from build123d import *

# Parameters (mm, degrees)
BASPROSKE_W         = 4.55
BASPROSKE_H         = 12
TOOTHCUT_DEPTH      = 18.569931702
TEETHCUTS_COUNT     = 22
TEETHCUTS_ANGLE     = 343.636363636
BORSKE_R            = 1.7
BORE_DEPTH          = 50.0000508
SKETCH1_R           = 5
BOSS_EXTRUDE1_DEPTH = 2
CUT_EXTRUDE1_START  = 2
SKETCH1_2_W         = 5
SKETCH1_2_H         = 5
CUT_EXTRUDE1_DEPTH  = 2.55
SKETCH1_4_R         = 6
SKETCH1_4_R_2       = 5
BOSS_EXTRUDE2_DEPTH = 1
CUT_EXTRUDE2_DEPTH  = 2


with BuildPart() as part:
    # BasProSke → Base-Revolve (revolve)
    with BuildSketch(Plane(origin=(0, 0, 0), x_dir=(1, 0, 0), z_dir=(0, 1, 0)), mode=Mode.PRIVATE) as base_revolve_sk:
        with Locations((2.275, 6)):
            Rectangle(BASPROSKE_W, BASPROSKE_H)
    revolve(base_revolve_sk.sketch.rotate(Axis((-10, 0, 0), (1, 0, 0)), 180), axis=Axis((-10, 0, 0), (1, 0, 0)))

    # TooCutSke → ToothCut (cut, through all)
    with BuildSketch(Plane(origin=(0, 0, 0), x_dir=(0, 0, -1), z_dir=(1, 0, 0))):
        with BuildLine():
            ThreePointArc((0.491001901, 9.736627657), (0, 9.749), (-0.491001901, 9.736627657))
            ThreePointArc((-0.491001901, 9.736627657), (-0.822824844, 10.904005344), (-1.46093845, 11.936327074))
            ThreePointArc((-1.46093845, 11.936327074), (0, 12.0254), (1.46093845, 11.936327074))
            ThreePointArc((1.46093845, 11.936327074), (0.822824844, 10.904005344), (0.491001901, 9.736627657))
        make_face()
    toothcut = extrude(amount=TOOTHCUT_DEPTH, mode=Mode.SUBTRACT)

    # TeethCuts: ToothCut ×22 about axis
    teethcuts_axis = Axis((-10, 0, 0), (1, 0, 0))
    for i in range(1, TEETHCUTS_COUNT):
        add(toothcut.rotate(teethcuts_axis, i * TEETHCUTS_ANGLE / (TEETHCUTS_COUNT - 1)), mode=Mode.SUBTRACT)

    # BorSke → Bore (cut, symmetric)
    with BuildSketch(Plane(origin=(0, 0, 0), x_dir=(0, 0, -1), z_dir=(1, 0, 0))):
        with Locations(Location((0, 0, 0), (0, 0, 180))):
            Circle(BORSKE_R)
    extrude(amount=BORE_DEPTH, both=True, mode=Mode.SUBTRACT)

    # Sketch1 → Boss-Extrude1 (add)
    with BuildSketch(Plane.ZY):
        with Locations(Location((0, 0, 0), (0, 0, 180))):
            Circle(SKETCH1_R)
    extrude(amount=BOSS_EXTRUDE1_DEPTH)

    # Sketch1<2> → Cut-Extrude1 (cut)
    with BuildSketch(Plane.ZY.offset(CUT_EXTRUDE1_START)):
        Rectangle(SKETCH1_2_W, SKETCH1_2_H)
    extrude(amount=-CUT_EXTRUDE1_DEPTH, mode=Mode.SUBTRACT)

    # Sketch1<4> → Boss-Extrude2 (add)
    with BuildSketch(Plane.ZY):
        with Locations(Location((0, 0, 0), (0, 0, 180))):
            Circle(SKETCH1_4_R)
        Circle(SKETCH1_4_R_2, mode=Mode.SUBTRACT)
    extrude(amount=BOSS_EXTRUDE2_DEPTH)

    # Sketch2 → Cut-Extrude2 (cut)
    with BuildSketch(Plane(origin=(4.55, 0, 0), x_dir=(0, 0, -1), z_dir=(1, 0, 0))):
        Polygon((1.645448267, 2.85), (-1.645448267, 2.85), (-3.290896534, 0), (-1.645448267, -2.85), (1.645448267, -2.85), (3.290896534, 0), align=None)
    extrude(amount=-CUT_EXTRUDE2_DEPTH, mode=Mode.SUBTRACT)


solid = part.part
Part model, mm, in its own coordinate system. A direction names the side the tool comes from. Round coordinates to 2 decimals unless told otherwise and drop trailing zeros. Loops run counter-clockwise (first coordinate to the right, second up) from the corner with the lowest first, then second, coordinate; pieces in that order, holes last. Notation, with made-up numbers: (62.25, 65.25) - (96.25, 65.25) arc R22 cw to (96.25, 73.25) - close; hole circle Ø6 at (30.5, -33.75). An arc over 180 degrees is marked (long way). Answer as a JSON object with one key per item and string values.
Item 1: Tool access for faces 1 (the face through (4, -2.85, 0)), 2 (the face through (2.24, -10.87, -0.81)), 3 (the face through (2.24, -1.38, 9.65)), 4 (the face through (2.2, -9.6, -5.2)), 5 (the face through (2.24, -7.76, -7.7)): list every direction of +Z, -Z, +X, -X, +Y, -Y with a clear straight run to the whole face (end or side of a thin tool).
Output:
{"face 1": "+X", "face 2": "+X, -X, -Y", "face 3": "+Z, +X, -X", "face 4": "+X, -X", "face 5": "-Z, +X, -X"}
Item 2: Band-saw the part on B-B on z = 10.75. List the corners of the cut face in (x, y).
Output:
{"outline": "(0, -3.76) - (4.55, -3.76) - (4.55, -2.41) - (0, -2.41) - close; (0, -0.78) - (4.55, -0.78) - (4.55, 0.78) - (0, 0.78) - close; (0, 2.41) - (4.55, 2.41) - (4.55, 3.76) - (0, 3.76) - close"}
Item 3: Wall check: L1, parallel to Y at x = 3.75, z = 10.75; L2, parallel to Y at x = 0.75, z = -9; L3, parallel to Z at x = 4, y = 9. Give the ranges that are in metal, low to high.
Output:
{"L1": "-3.76 to -2.41, -0.78 to 0.78, 2.41 to 3.76", "L2": "-6.58 to -4.74, -3.75 to 3.75, 4.74 to 6.58", "L3": "-7.94 to -7.06, -5.06 to 5.06, 7.06 to 7.94"}
Item 4: Pull direction Y, two halves, no side cores. Call faces 6 (the face through (2.24, 8.73, -6.59)), 7 (the face through (2.2, -9.6, 5.2)), 8 (the face through (2.24, -8.71, -6.56)): pulls with the +Y half, pulls with the -Y half, needs draft (parallel to the pull), parting line crosses it, or undercut.
Output:
{"face 6": "pulls with the +Y half", "face 7": "undercut", "face 8": "pulls with the -Y half"}
Item 5: Band-saw the part on A-A on z = 0. List the corners of the cut face in (x, y), plus the area to 3 significant figures.
Output:
{"outline": "(-2, -5) - (-1, -5) - (-1, -6) - (0, -6) - (0, -9.75) - (4.55, -9.75) - (4.55, -2.85) - (2.55, -2.85) - (2.55, -1.7) - (0.55, -1.7) - (0.55, -2.5) - (-2, -2.5) - close; (-2, 2.5) - (0.55, 2.5) - (0.55, 1.7) - (2.55, 1.7) - (2.55, 2.85) - (4.55, 2.85) - (4.55, 9.75) - (0, 9.75) - (0, 6) - (-1, 6) - (-1, 5) - (-2, 5) - close", "area": "79.8 mm2"}
Item 6: Pin check, flat tips, straight feed: pin 1 (2 mm diameter, centred on x = -0.5, z = -0.5, fed in from +Y); pin 2 (1 mm diameter, centred on x = 0, y = -6.5, fed in from +Z); pin 3 (1.5 mm diameter, centred on y = -1, z = -0.5, fed in from -X); pin 4 (2.5 mm diameter, centred on y = 0, z = 0, fed in from +X). Stop position of each tip, or through.
Output:
{"pin 1": "y = 11.82", "pin 2": "z = 10.24", "pin 3": "x = 0.55", "pin 4": "through"}
